Work out the finished part from the listing and answer in its coordinate system (mm). A direction names the side the tool comes from. Round coordinates to 2 decimals unless told otherwise and drop trailing zeros. Order: outer loops, then holes, each group sorted by start corner. A loop starts at its lowest first (then second) coordinate and runs counter-clockwise, first axis right, second up. Notation, with made-up numbers: (70, -31.75) - (78, -31.75) arc R23 ccw to (78, -17.75) - close; hole circle Ø3 at (-19.5, 54.5). An arc over 180 degrees is marked (long way). Use one line per item in the form item = value. Start each with the question number.
Q1. For a pull along X with two mould halves and no side action, classify faces 4 (the flat face through (-1, 1, -3)), 5 (the flat face through (70, 2, 0)), 6 (the flat face through (-67, 2, 1.5)) as +X half, -X half, draft (parallel to the pull), parting line (faces both ways), or undercut.
Q2. Find the intervals of material crossed by line 1 (X direction, y = 2.65, z = 2.2); line 2 (Z direction, x = 49, y = 1.2); line 3 (X direction, y = 1.3, z = 0.5), in increasing order. Write a range as [from, to].
Q3. Given P1, Ø3, axis at x = -18, z = 1, coming from the -Y side; P2, Ø1.5, axis at x = 67.5, y = 1, coming from the -Z side; P3, Ø1.5, axis at x = -66.5, y = 2, coming from the +Z side, each flat-ended and moving along its own axis, determine where each tip first touches the part or whether it passes through.
Q4. Which of the six approach directions +Z, -Z, +X, -X, +Y, -Y give full straight-line access (tool end or side, diameter ignored) to faces 1 (the flat face through (-67, 2, -1.5)), 2 (the flat face through (67, 2, 1.5)), 3 (the flat face through (1, 3, 0))?
Q5. The part is cut by section A-A on z = 0. Determine the outline of the cut face in (x, y) (3 decimals).
Q6. The part is cut by section B-B on y = 0.55. Determine the outline of the cut face in (x, z) (3 decimals), plus the area to 3 significant figures.
from build123d import *

# Parameters (mm, degrees)
SKETCH1_W               = 137
SKETCH1_H               = 6
BOSS_EXTRUDE1_DEPTH     = 3
SKETCH2_W               = 3
SKETCH2_H               = 1.5
CUT_EXTRUDE1_DEPTH      = 3
MIRROR2_COPY_1_SKETCH_W = 3
MIRROR2_COPY_1_SKETCH_H = 1.5
MIRROR2_COPY_1_DEPTH    = 3
BOSS_EXTRUDE2_DEPTH     = 3
CUT_EXTRUDE2_DEPTH      = 3


with BuildPart() as part:
    # Sketch1 → Boss-Extrude1 (new body)
    with BuildSketch(Plane(origin=(0, 0, 0), x_dir=(1, 0, 0), z_dir=(0, 1, 0))):
        Rectangle(SKETCH1_W, SKETCH1_H)
    extrude(amount=BOSS_EXTRUDE1_DEPTH)

    # Sketch2 → Cut-Extrude1 (cut)
    with BuildSketch(Plane(origin=(0, 3, 0), x_dir=(1, 0, 0), z_dir=(0, 1, 0))):
        with Locations((67, 2.25)):
            Rectangle(SKETCH2_W, SKETCH2_H)
    cut_extrude1 = extrude(amount=-CUT_EXTRUDE1_DEPTH, mode=Mode.SUBTRACT)

    # Mirror1: Cut-Extrude1 across plane
    add(cut_extrude1.mirror(Plane.XY), mode=Mode.SUBTRACT)

    # Mirror2: Cut-Extrude1 across plane
    add(cut_extrude1.mirror(Plane(origin=(0, 0, 0), x_dir=(0, 0, 1), z_dir=(1, 0, 0))), mode=Mode.SUBTRACT)

    # Mirror2 copy 1 sketch → Mirror2 copy 1 (cut)
    with BuildSketch(Plane(origin=(0, 3, 0), x_dir=(-1, 0, 0), z_dir=(0, 1, 0))):
        with Locations((67, 2.25)):
            Rectangle(MIRROR2_COPY_1_SKETCH_W, MIRROR2_COPY_1_SKETCH_H)
    extrude(amount=-MIRROR2_COPY_1_DEPTH, mode=Mode.SUBTRACT)

    # Sketch3 → Boss-Extrude2 (add)
    with BuildSketch(Plane(origin=(0, 3, 0), x_dir=(1, 0, 0), z_dir=(0, 1, 0))):
        Polygon((70, 3), (68.5, 3), (68.5, 1.5), (68.5, -1.5), (68.5, -3), (70, -3), align=None)
    boss_extrude2 = extrude(amount=-BOSS_EXTRUDE2_DEPTH)

    # Mirror3: Boss-Extrude2 across plane
    add(boss_extrude2.mirror(Plane(origin=(0, 0, 0), x_dir=(0, 0, 1), z_dir=(1, 0, 0))))

    # Sketch4 → Cut-Extrude2 (cut)
    with BuildSketch(Plane(origin=(0, 3, 0), x_dir=(1, 0, 0), z_dir=(0, 1, 0))):
        with BuildLine():
            ThreePointArc((-50.125, 0), (-49.125, -1), (-48.125, 0))
            Line((-48.125, 0), (-50.125, 0))
        make_face()
        with BuildLine():
            Line((-50.125, 0), (-48.125, 0))
            ThreePointArc((-48.125, 0), (-49.125, 1), (-50.125, 0))
        make_face()
        with BuildLine():
            ThreePointArc((-15.375, 0), (-16.375, 1), (-17.375, 0))
            Line((-17.375, 0), (-15.375, 0))
        make_face()
        with BuildLine():
            Line((-15.375, 0), (-17.375, 0))
            ThreePointArc((-17.375, 0), (-16.375, -1), (-15.375, 0))
        make_face()
    cut_extrude2 = extrude(amount=-CUT_EXTRUDE2_DEPTH, mode=Mode.SUBTRACT)

    # Mirror4: Cut-Extrude2 across plane
    add(cut_extrude2.mirror(Plane(origin=(0, 0, 0), x_dir=(0, 0, 1), z_dir=(1, 0, 0))), mode=Mode.SUBTRACT)


solid = part.part
Found:
q1.face_4 = draft
q1.face_5 = +X half
q1.face_6 = undercut
q2.line_1 = [-70, -68.5], [-65.5, 65.5], [68.5, 70]
q2.line_2 = [-3, -0.99], [0.99, 3]
q2.line_3 = [-70, -49.99], [-48.26, -17.24], [-15.51, 15.51], [17.24, 48.26], [49.99, 70]
q3.P1 = 0
q3.P2 = -1.5
q3.P3 = 1.5
q4.face_1 = -Z, +Y, -Y
q4.face_2 = +Z, +Y, -Y
q4.face_3 = +Z, -Z, +X, -X, +Y
q5.outline = (-70, 0) - (-50.125, 0) - (-50.125, 3) - (-70, 3) - close; (-48.125, 0) - (-17.375, 0) - (-17.375, 3) - (-48.125, 3) - close; (-15.375, 0) - (15.375, 0) - (15.375, 3) - (-15.375, 3) - close; (17.375, 0) - (48.125, 0) - (48.125, 3) - (17.375, 3) - close; (50.125, 0) - (70, 0) - (70, 3) - (50.125, 3) - close
q6.outline = (-70, -3) - (-68.5, -3) - (-68.5, -1.5) - (-65.5, -1.5) - (-65.5, -3) - (65.5, -3) - (65.5, -1.5) - (68.5, -1.5) - (68.5, -3) - (70, -3) - (70, 3) - (68.5, 3) - (68.5, 1.5) - (65.5, 1.5) - (65.5, 3) - (-65.5, 3) - (-65.5, 1.5) - (-68.5, 1.5) - (-68.5, 3) - (-70, 3) - close; hole circle Ø2 at (-49.125, 0); hole circle Ø2 at (-16.375, 0); hole circle Ø2 at (16.375, 0); hole circle Ø2 at (49.125, 0)
q6.area = 809 mm²
